```python
from build123d import *

# Parameters (mm, degrees)
SKETCH1_R           = 4.05
BOSS_EXTRUDE1_DEPTH = 0.9
CUT_EXTRUDE1_START  = -0.9
CUT_EXTRUDE1_DEPTH  = 0.9
SKETCH3_R           = 2.5
BOSS_EXTRUDE2_DEPTH = 3
CUT_EXTRUDE3_DEPTH  = 2.5
CUT_EXTRUDE4_DEPTH  = 0.25


with BuildPart() as part:
    # Sketch1 → Boss-Extrude1 (new body)
    with BuildSketch(Plane(origin=(0, 0, 0), x_dir=(1, 0, 0), z_dir=(0, 1, 0))):
        with Locations(Location((0, 0, 0), (0, 0, 270))):
            Circle(SKETCH1_R)
    extrude(amount=BOSS_EXTRUDE1_DEPTH)

    # Sketch2 → Cut-Extrude1 (cut)
    with BuildSketch(Plane(origin=(0, 0.9, 0), x_dir=(1, 0, 0), z_dir=(0, 1, 0)).offset(CUT_EXTRUDE1_START)):
        with BuildLine():
            Line((3.75, 1.529705854), (3.75, 0))
            Line((3.75, 0), (3.75, -1.529705854))
            ThreePointArc((3.75, -1.529705854), (3.97429239, -0.779422863), (4.05, 0))
            ThreePointArc((4.05, 0), (3.97429239, 0.779422863), (3.75, 1.529705854))
        make_face()
    extrude(amount=CUT_EXTRUDE1_DEPTH, mode=Mode.SUBTRACT)

    # Sketch3 → Boss-Extrude2 (add)
    with BuildSketch(Plane(origin=(0, 0.9, 0), x_dir=(1, 0, 0), z_dir=(0, 1, 0))):
        with Locations(Location((0, 0, 0), (0, 0, 270))):
            Circle(SKETCH3_R)
    extrude(amount=BOSS_EXTRUDE2_DEPTH)

    # Sketch4 → Cut-Extrude3 (cut)
    with BuildSketch(Plane.XZ):
        with BuildLine():
            Line((-1.984313483, 0.25), (-0.25, 0.25))
            Line((-0.25, 0.25), (-0.25, 1.984313483))
            ThreePointArc((-0.25, 1.984313483), (-1.414213562, 1.414213562), (-1.984313483, 0.25))
        make_face()
        with BuildLine():
            Line((0.25, 1.984313483), (0.25, 0.25))
            Line((0.25, 0.25), (1.984313483, 0.25))
            ThreePointArc((1.984313483, 0.25), (1.414213562, 1.414213562), (0.25, 1.984313483))
        make_face()
        with BuildLine():
            Line((-0.25, -1.984313483), (-0.25, -0.25))
            Line((-0.25, -0.25), (-1.984313483, -0.25))
            ThreePointArc((-1.984313483, -0.25), (-1.414213562, -1.414213562), (-0.25, -1.984313483))
        make_face()
    extrude(amount=-CUT_EXTRUDE3_DEPTH, mode=Mode.SUBTRACT)

    # Sketch4_3 → Cut-Extrude4 (cut)
    with BuildSketch(Plane.XZ):
        with BuildLine():
            Line((1.984313483, -0.25), (0.25, -0.25))
            Line((0.25, -0.25), (0.25, -1.984313483))
            ThreePointArc((0.25, -1.984313483), (1.414213562, -1.414213562), (1.984313483, -0.25))
        make_face()
    extrude(amount=-CUT_EXTRUDE4_DEPTH, mode=Mode.SUBTRACT)


solid = part.part
```
Geometry check sheet. Reference: the model listing, model coordinates, mm. A direction names the side the tool comes from. Coordinates: 2 decimals unless noted, no trailing zeros. Write each loop counter-clockwise with the first axis right and the second up, starting at its lowest first coordinate (ties: lowest second). Pieces come first, ordered by that corner, then holes. Notation, with made-up numbers: M 24,11 L 59,11 A7 cw 59,23 Z; hole C 52.5,57 d8. An arc over 180 degrees is marked long. Use one line per item in the form item = value. Start each with the question number.
1) Section check D-D on y = 0.6. Enter the section's corners in (x, z).
2) Thickness scan on probe 1 along Z at (x, y) = (-1, 2.45); probe 2 along X at (y, z) = (1.05, 1.75). Record the ranges inside material, lowest first. Write a range as from..to.
3) Set-up check for faces 5 (the flat face through (-1, 1, 0.25)), 6 (the flat face through (3.75, 0.4, 0)), 7 (the flat face through (-2, 0.9, 2)): record each of +Z, -Z, +X, -X, +Y, -Y from which the full face is reachable in a straight line by a thin tool's end or side.
4) Section check B-B on z = 0. Enter the section's corners in (x, y).
5) Go/stop test with flat-tipped pins: pin 1 Ø1.5 at (y, z) = (3, -2.5) entering from +X; pin 2 Ø0.5 at (x, y) = (-1, 2) entering from -Z; pin 3 Ø0.5 at (x, z) = (-1, -1) entering from -Y. Record where each tip stops, or that it passes through.
6) Section check C-C on x = 0. Enter the section's corners in (y, z).
7) Section check A-A on y = 1.5. Enter the section's corners in (x, z).
8) Release check for a two-part mould opening along Z. For faces 1 (the flat face through (1, 0.25, -1)), 2 (the cylindrical face through (-2.44, 2.38, -0.54)), 3 (the flat face through (-1, 2.5, -1)), 4 (the flat face through (0, 0, 0)) record: pulls with the +Z half, pulls with the -Z half, needs draft (parallel to the pull), parting line crosses it, or undercut.
Responses:
q1.outline = M 3.75,-1.53 L 3.75,1.53 A4.05 ccw long Z; hole M -1.98,-0.25 A2 ccw -0.25,-1.98 L -0.25,-0.25 Z; hole M -1.98,0.25 L -0.25,0.25 L -0.25,1.98 A2 ccw Z; hole M 0.25,0.25 L 1.98,0.25 A2 ccw 0.25,1.98 Z
q2.probe_1 = -2.29..-1.73, -0.25..0.25, 1.73..2.29
q2.probe_2 = -1.79..-0.97, -0.25..0.25, 0.97..1.79
q3.face_5 = -Y
q3.face_6 = +Z, -Z, +X, +Y, -Y
q3.face_7 = +Y
q4.outline = M -4.05,0 L 3.75,0 L 3.75,0.9 L 2.5,0.9 L 2.5,3.9 L -2.5,3.9 L -2.5,0.9 L -4.05,0.9 Z
q5.pin_1 = 1.79
q5.pin_2 = -2.38
q5.pin_3 = 2.5
q6.outline = M 0,-4.05 L 0.9,-4.05 L 0.9,-2.5 L 3.9,-2.5 L 3.9,2.5 L 0.9,2.5 L 0.9,4.05 L 0,4.05 Z
q7.outline = C 0,0 d5; hole M -1.98,-0.25 A2 ccw -0.25,-1.98 L -0.25,-0.25 Z; hole M -1.98,0.25 L -0.25,0.25 L -0.25,1.98 A2 ccw Z; hole M 0.25,0.25 L 1.98,0.25 A2 ccw 0.25,1.98 Z
q8.face_1 = undercut
q8.face_2 = parting line crosses it
q8.face_3 = undercut
q8.face_4 = needs draft
